Geometry: final body of the model. Coordinates: model frame, mm. Face numbers are marked on the shaded views. Give positions to 0.01 mm unless a question says otherwise; leave off trailing zeros. Loops run counter-clockwise (first coordinate to the right, second up) from the corner with the lowest first, then second, coordinate; pieces in that order, holes last.
from build123d import *

# Parameters (mm, degrees)
PAD_DEPTH   = 30
FILLET_R    = 4
FILLET001_R = 4


with BuildPart() as part:
    # Sketch → Pad (new body, symmetric)
    with BuildSketch(Plane.YZ):
        with BuildLine():
            Line((-30.928615, 0), (-20.928615, 0))
            Line((-20.928615, 0), (-0.928621, 40.000014))
            Line((-0.928621, 40.000014), (5.816401, 53.490069))
            ThreePointArc((5.816401, 53.490069), (8.759064, 25.831927), (19.071385, 7e-06))
            Line((19.071385, 7e-06), (29.071385, 7e-06))
            ThreePointArc((29.907603, 101.672508), (15.589377, 50.95058), (29.071385, 7e-06))
            Line((19.907603, 101.672508), (29.907603, 101.672508))
            Line((-0.928626, 60.00002), (19.907603, 101.672508))
            Line((-0.928626, 60.00002), (-26.903694, 8.049846))
            Line((-39.425677, 14.310833), (-26.903694, 8.049846))
            Line((-37.18961, 18.782969), (-39.425677, 14.310833))
            Line((-42.556174, 21.466249), (-37.18961, 18.782969))
            Line((-45.905216, 14.768161), (-42.556174, 21.466249))
            ThreePointArc((-45.905216, 14.768161), (-46.258493, 9.797157), (-42.993266, 6.032322))
            Line((-30.928615, 0), (-42.993266, 6.032322))
        make_face()
    extrude(amount=PAD_DEPTH, both=True)

    # Fillet
    fillet_edges = [part.edges().sort_by_distance(p)[0] for p in [
        (0, -37.18961, 18.782969),
    ]]
    fillet(fillet_edges, radius=FILLET_R)

    # Fillet001
    fillet001_edges = [part.edges().sort_by_distance(p)[0] for p in [
        (0, -20.928615, 0),
    ]]
    fillet(fillet001_edges, radius=FILLET001_R)


solid = part.part
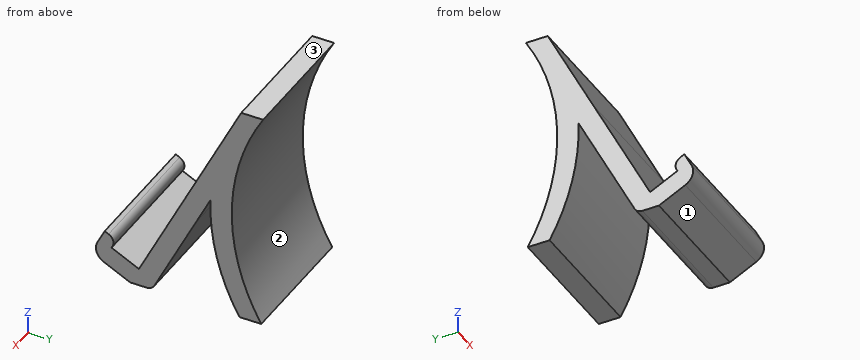
Item 1: Pin query (flat end, axial travel): pin 1 (2 mm diameter, centred on x = 15, z = 51.5, fed in from +Y); pin 2 (4 mm diameter, centred on x = 13, z = 51, fed in from -Y); pin 3 (10 mm diameter, centred on x = 18.5, z = 53.5, fed in from +Y). Return the tip coordinate at first contact, or that it passes through.
Values follow:
pin 1: stops at y = 15.61
pin 2: stops at y = -6.43
pin 3: stops at y = 15.94
Item 2: Ray query, probe 1 along Y at (x, z) = (-19, 15); probe 2 along Y at (x, z) = (-24, 8.5); probe 3 along Z at (x, y) = (6, 24). Return the intervals inside material, ascending.
Values follow:
probe 1: y = -45.79 to -39.08, -23.43 to -13.43, 12.09 to 21.97
probe 2: y = -45.66 to -27.8, -26.68 to -16.68, 14.75 to 24.67
probe 3: z = 0 to 10, 90.26 to 101.67
Item 3: Section query C-C on z = 28. Return loops of the section in (x, y).
Values follow:
outline: (-30, -16.93) - (30, -16.93) - (30, -6.93) - (-30, -6.93) - close; (-30, 8.25) - (30, 8.25) - (30, 18.07) - (-30, 18.07) - close
Item 4: Section query A-A on z = 42. Return loops of the section in (x, y), plus the area to 3 significant figures.
Values follow:
outline: (-30, -9.93) - (30, -9.93) - (30, 0.07) - (-30, 0.07) - close; (-30, 6.11) - (30, 6.11) - (30, 15.92) - (-30, 15.92) - close
area: 1,190 mm2
Item 5: Draft query along Z for the marked faces 1, 2 and 3. Return one class per face: +Z half, -Z half, draft (parallel to the pull), parting line (faces both ways), or undercut.
Values follow:
face 1: -Z half
face 2: undercut
face 3: +Z half
Item 6: Section query B-B on x = -23.5. Return loops of the section in (y, z), plus the area to 3 significant figures.
Values follow:
outline: (-45.91, 14.77) arc R6.51 ccw to (-42.99, 6.03) - (-30.93, 0) - (-23.4, 0) arc R4 ccw to (-19.82, 2.21) - (5.82, 53.49) arc R101.89 ccw to (19.07, 0) - (29.07, 0) arc R99.91 cw to (29.91, 101.67) - (19.91, 101.67) - (-26.9, 8.05) - (-39.43, 14.31) - (-38.98, 15.21) arc R4 ccw to (-40.77, 20.57) - (-42.56, 21.47) - close
area: 1,870 mm2
Item 7: Section query D-D on y = 9.5. Return loops of the section in (x, z) (3 decimals), plus the area to 3 significant figures.
Values follow:
outline: (-30, 23.015) - (30, 23.015) - (30, 80.857) - (-30, 80.857) - close
area: 3,470 mm2
